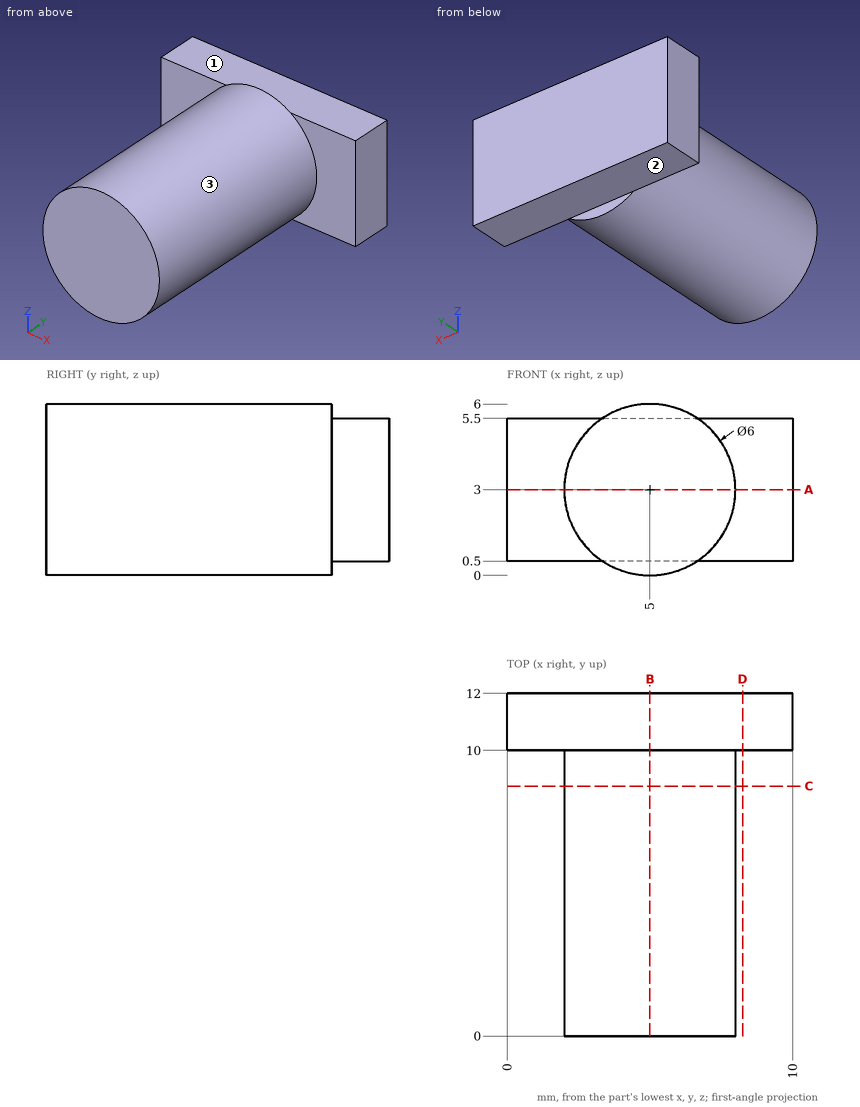
Source: three-view drawing plus pictorial views. Frame: mm from the lowest corner of the part. A direction names the side the tool comes from. Coordinates: 2 decimals unless noted, no trailing zeros. Order: outer loops, then holes, each group sorted by start corner. A loop starts at its lowest first (then second) coordinate and runs counter-clockwise, first axis right, second up.
Item 1: Cut plane B-B (x = 5). Return loops of the section in (y, z), plus the area to 3 significant figures.
Output values:
outline: (0, 0) - (10, 0) - (10, 0.5) - (12, 0.5) - (12, 5.5) - (10, 5.5) - (10, 6) - (0, 6) - close
area: 70.0 mm2
Item 2: Cut plane D-D (x = 8.25). Return loops of the section in (y, z).
Output values:
outline: (10, 0.5) - (12, 0.5) - (12, 5.5) - (10, 5.5) - close
Item 3: Set-up query: the marked faces 1, 2 and 3. Return all of +Z, -Z, +X, -X, +Y, -Y with unobstructed straight access to the full face (end or side cutting, diameter ignored); none if empty.
Output values:
face 1: +Z, +X, -X, +Y
face 2: -Z, +X, -X, +Y
face 3: -Y
Item 4: First-contact query: P1, Ø3, axis at y = 7, z = 4.5, coming from the -X side; P2, Ø3, axis at x = 4.5, y = 3, coming from the +Z side; P3, Ø1.5, axis at y = 9, z = 1.5, coming from the +X side; P4, Ø1, axis at x = 3, y = 11, coming from the +Z side. Flat tips, straight axial feed; report the tip coordinate or a pass-through.
Output values:
P1: stops at x = 2
P2: stops at z = 6
P3: stops at x = 7.9
P4: stops at z = 5.5
Item 5: Material intervals for line 1 (Y direction, x = 1.75, z = 5.45); line 2 (Y direction, x = 6, z = 5.6); line 3 (X direction, y = 5.25, z = 3.05), sorted ascending.
Output values:
line 1: y = 10 to 12
line 2: y = 0 to 10
line 3: x = 2 to 8
Item 6: Cut plane C-C (y = 8.75). Return loops of the section in (x, z).
Output values:
outline: circle Ø6 at (5, 3)
Item 7: Cut plane A-A (z = 3). Return loops of the section in (x, y), plus the area to 3 significant figures.
Output values:
outline: (0, 10) - (2, 10) - (2, 0) - (8, 0) - (8, 10) - (10, 10) - (10, 12) - (0, 12) - close
area: 80.0 mm2
